Autodesk Inventor part; units mm, degrees
ref_plane "YZ Plane" through (0, 0, 0) normal (1, 0, 0) x (0, 1, 0)
ref_plane "XZ Plane" through (0, 0, 0) normal (0, 1, 0) x (-1, 0, 0)
ref_plane "XY Plane" through (0, 0, 0) normal (0, 0, 1) x (1, 0, 0)
sketch "スケッチ1" plane through (0, 0, 0) normal (0, 0, 1) x (1, 0, 0)
  line L0 (0, 0) -> (6, 0) construction
  line L1 (0, -3.25) -> (6, -3.25)
  line L2 (6, 3.25) -> (0, 3.25)
  arc A0 (0, 3.25) -> (0, -3.25) centre (0, 0) ccw
  arc A1 (6, -3.25) -> (6, 3.25) centre (6, 0) ccw
  line L3 (-15, 0) -> (-9, 0) construction
  line L4 (-9, 3.25) -> (-15, 3.25)
  arc A2 (-15, 3.25) -> (-18.25, 0) centre (-15, 0) ccw
  arc A3 (-9, -3.25) -> (-9, 3.25) centre (-9, 0) ccw
  line L5 (-9, 0) -> (0, 0)
  circle A4 centre (-15, 0) radius 3.25 construction
  circle A5 centre (2.604723, -14.772116) radius 3.25
  line L6 (0, 0) -> (2.604723, -14.772116) construction
  arc A6 (-11.29159, -3.25) -> (2.040366, -11.571491) centre (0, 0) ccw
  line L7 (0, 0) -> (125.4, 0)
  line L8 (125.340198, -9.986176) -> (5.767236, -15.521122)
  line L9 (-11.29159, -3.25) -> (-9, -3.25)
  arc A7 (-13.5, 8.25) -> (-15, 6.75) centre (-15, 8.25) ccw
  line L10 (-15, 8.25) -> (-15, 6.75) construction
  line L11 (-15, 3.25) -> (-18.25, 3.25)
  line L12 (-18.25, 3.25) -> (-18.25, 8.25)
  line L13 (-13.5, 8.25) -> (-11.75, 8.25)
  line L14 (-15, 6.75) -> (-9.617692, 6.75)
  arc A8 (-11.75, 0) -> (-11.29159, -3.25) centre (0, 0) ccw
  arc A9 (2.040366, -11.571491) -> (-11.75, 0) centre (0, 0) ccw construction
  line L15 (9.617692, 6.75) -> (125.4, 0)
  line L16 (-9.617692, 6.75) -> (9.617692, 6.75)
  line L17 (-15, 6.75) -> (-15, 0) construction
  arc A10 (-11.75, 8.25) -> (-18.25, 8.25) centre (-15, 8.25) ccw
  circle A11 centre (125.108999, -4.991525) radius 5
  point P0 (3, 0)
  point P1 (-12, 0)
  point P2 (2.040366, -11.571491)
  point P3 (124.817998, 0)
  dimension "d6" = 6.5
  dimension "d7" = 6.5
  dimension "d0" = 6.5
  dimension "d1" = 6
  dimension "d3" = 6.5
  dimension "d4" = 6
  dimension "d5" = 15
  dimension "d8" = 15
  dimension "d9" = 100
  dimension "d11" = 125.4
  dimension "d12" = 3
  dimension "d13" = 5
  dimension "d14" = 3.25
  dimension "d15" = 6.5
  dimension "d18" = 10
extrude "押し出し1" add sketch "スケッチ1" along normal blind 5 contours L1 A1 L7 A11 L8 A5 A6 L9 A3 L5 A0 | L5 A3 L4 L11 L12 A10 L13 A7 L14 L16 L15 A11 L7 A1 L2 A0 | L7 A11 picked at (123.673178, -4.767327)
sketch "スケッチ2" plane through (0, 0, 5) normal (0, 0, 1) x (1, 0, 0)
  arc A0 (-15, 6.75) -> (-13.5, 8.25) centre (-15, 8.25) ccw
  line L0 (-13.5, 8.25) -> (-11.75, 8.25)
  arc A1 (-11.75, 8.25) -> (-18.25, 8.25) centre (-15, 8.25) ccw
  line L1 (-18.25, 8.25) -> (-18.25, 3.25)
  arc A2 (-9, 3.25) -> (-9, -3.25) centre (-9, 0) ccw
  line L2 (-9, -3.25) -> (-11.29159, -3.25)
  arc A3 (-11.29159, -3.25) -> (2.040366, -11.571491) centre (0, 0) ccw
  arc A4 (2.040366, -11.571491) -> (5.767236, -15.521122) centre (2.604723, -14.772116) ccw
  line L3 (5.767236, -15.521122) -> (125.340198, -9.986176)
  arc A5 (125.340198, -9.986176) -> (125.4, 0) centre (125.108999, -4.991525) ccw
  line L4 (125.4, 0) -> (124.817998, 0)
  line L5 (124.817998, 0) -> (125.4, 0)
  line L6 (125.4, 0) -> (9.617692, 6.75)
  line L7 (0, 3.25) -> (6, 3.25)
  arc A6 (6, 3.25) -> (6, -3.25) centre (6, 0) ccw
  line L8 (6, -3.25) -> (0, -3.25)
  arc A7 (0, -3.25) -> (0, 3.25) centre (0, 0) ccw
  arc A8 (125.224598, -7.488851) -> (125.202485, -2.493273) centre (125.108999, -4.991525) ccw
  line L9 (125.224598, -7.488851) -> (8.045869, -12.912969)
  arc A9 (8.045869, -12.912969) -> (1.606246, -9.109472) centre (2.604723, -14.772116) ccw
  arc A10 (-7.416667, -5.527708) -> (1.606246, -9.109472) centre (0, 0) ccw
  arc A11 (-7.416667, -5.527708) -> (-9, 5.75) centre (-9, 0) ccw
  line L10 (125.254499, -2.495762) -> (9.041316, 4.279357)
  line L11 (6, 5.25) -> (0, 5.25)
  arc A12 (0, 5.25) -> (0, -5.25) centre (0, 0) ccw
  line L12 (0, -5.25) -> (6, -5.25)
  arc A13 (6, -5.25) -> (6, 5.25) centre (6, 0) ccw
  point P0 (-4.194444, -3.157394)
  point P1 (125.254499, -2.495762)
  point P2 (9.678702, 3.745617)
  point P3 (-4.194444, 3.157394)
  dimension "d19" = 2.5
  dimension "d20" = 2.5
  dimension "d21" = 2
extrude "押し出し2" cut sketch "スケッチ2" against normal blind 4 contours L9 A9 A10 A11 A12 L12 A13 L10 A8
fillet "フィレット1" radius 1.05 4 edges at (8.0459, -12.913, 3) (-7.4167, -5.5277, 3) (-4.1944, -3.1574, 3) (9.0413, 4.2794, 3)
properties part number "ウィング" material "ポリカーボネート、クリア"
CAD build for the part. Positions are in the model's coordinates, mm. A direction names the side the tool comes from. Give positions to 0.01 mm unless a question says otherwise; leave off trailing zeros. Order: outer loops, then holes, each group sorted by start corner. A loop starts at its lowest first (then second) coordinate and runs counter-clockwise, first axis right, second up. Notation, with made-up numbers: M 44.25,73 L 73.25,73 A29 cw 73.25,111 Z; hole C 68.5,-11 d9. An arc over 180 degrees is marked long. Put each result on its own line as item: value. Start each with the question number.
(1) Which spindle directions (+Z, -Z, +X, -X, +Y, -Y) get a long thin tool onto all of the face, cutting with end or side? Do faces 1 (the cylindrical face through (10.49, -2.72, 3.03)), 2 (the flat face through (-14, 3.25, 2)), 3 (the cylindrical face through (9.25, 0.07, 2.46)), 4 (the flat face through (66.698, 3.422, 2.465)). Say none if no direction does.
(2) Saw through at A-A, the plane x = 112.5. Write the cut outline in (y, z), then the cut area to 3 significant figures.
(3) Saw through at C-C, the plane x = 76. Write the cut outline in (y, z).
(4) Flat gauge pins, fed straight in: pin 1 Ø1 at (x, y) = (3.5, -7.5) entering from +Z; pin 2 Ø2.5 at (x, z) = (-12, 2) entering from -Y; pin 3 Ø1.2 at (x, z) = (4, 2.5) entering from -Y. Where does each tip first touch, or does it go through?
(5) Mould opens along X. For faces 5 (the cylindrical face through (-15.1, 11.5, 2.5)), 6 (the cylindrical face through (-2.74, -8.835, 3.028)), 7 (the flat face through (66.391, -12.715, 2.465)) say: +X half, -X half, draft (parallel to the pull), parting line (faces both ways), or undercut.
(6) Drill centre lines: line 1 along Y through (x, z) = (8, 3.3); line 2 along X through (y, z) = (-4, 1.4); line 3 along X through (y, z) = (-4.75, 4.55). Where is each one in solid material? Low to high.
Check result:
1. face 1: +Z
1. face 2: +Z, -Z, -X
1. face 3: +Z, -Z
1. face 4: +Z, -Z, +X, +Y
2. outline: M -10.58,0 L 0.75,0 L 0.75,5 L -1.75,5 L -1.75,1 L -8.08,1 L -8.08,5 L -10.58,5 Z
2. area: 31.4 mm2
3. outline: M -12.27,0 L 2.88,0 L 2.88,5 L 0.38,5 L 0.38,1 L -9.77,1 L -9.77,5 L -12.27,5 Z
4. pin 1: stops at z = 1
4. pin 2: stops at y = -4.74
4. pin 3: stops at y = -12.21
5. face 5: parting line
5. face 6: undercut
5. face 7: +X half
6. line 1: y = -15.42 to -12.58, -4.85 to -2.56, 2.56 to 6.75
6. line 2: x = -11.05 to -4.87, -3.4 to 9.4, 127.4 to 130.01
6. line 3: x = -10.75 to -5.76, -2.24 to 8.24, 127.6 to 130.1
